Check sheet for the modelled part. Datum: model origin and axes. Units: mm. Face numbers are marked on the shaded views. A direction names the side the tool comes from. Round coordinates to 2 decimals unless told otherwise and drop trailing zeros. Write each loop counter-clockwise with the first axis right and the second up, starting at its lowest first coordinate (ties: lowest second). Pieces come first, ordered by that corner, then holes.
Item 1: Section check B-B, the plane z = 6.5. Record the cut outline in (x, y) (3 decimals), plus the area to 3 significant figures.
Item 2: Depth check by flat-ended pin: pin 1 (8 mm diameter, centred on y = 4, z = 5, fed in from +X) (3 decimals); pin 2 (1.5 mm diameter, centred on y = 15, z = 29, fed in from -X); pin 3 (2 mm diameter, centred on x = 37, z = 50, fed in from +Y). Enter the tip coordinate at first touch or a pass-through.
Item 3: Release check for a two-part mould opening along X. For the marked faces 5, 6 and 7 record: pulls with the +X half, pulls with the -X half, needs draft (parallel to the pull), parting line crosses it, or undercut.
Item 4: Section check D-D, the plane z = 18.5. Record the cut outline in (x, y) (3 decimals).
Item 5: Section check A-A, the plane y = 18. Record the cut outline in (x, z) (3 decimals).
Item 6: Set-up check for the marked faces 1, 2, 3 and 4: record each of +Z, -Z, +X, -X, +Y, -Y from which the full face is reachable in a straight line by a thin tool's end or side.
Item 7: Section check C-C, the plane x = 25. Record the cut outline in (y, z) (3 decimals).
Item 8: Material ranges on line 1 along Y through (x, z) = (68.5, 54); line 2 along Z through (x, y) = (5, 7.5) (3 decimals); line 3 along X through (y, z) = (2, 10) (3 decimals), recorded low to high.
from build123d import *

# Parameters (mm, degrees)
F1_DEPTH = 63.5
F2_DEPTH = 25.4


with BuildPart() as f1:
    # F0 (on Front) → F1 (new body, symmetric)
    with BuildSketch(Plane.XZ):
        Polygon((41.275, -9.525), (41.275, 9.525), (22.225, 9.525), (-41.275, 9.525), (-41.275, -9.525), align=None)
    extrude(amount=F1_DEPTH, both=True)

    # F0 (on Front) → F2 (join, symmetric)
    with BuildSketch(Plane.XZ):
        Polygon((60.325, 61.9252), (60.325, 42.8752), (60.325, 38.1), (85.725, 38.1), (85.547439, 66.675), (60.325, 66.675), align=None)
        with BuildLine():
            Line((22.225, 9.525), (41.275, 9.525))
            Line((41.275, 9.525), (41.275, 27.0002))
            ThreePointArc((41.275, 27.0002), (45.92468, 38.22552), (57.15, 42.8752))
            Line((57.15, 42.8752), (60.325, 42.8752))
            Line((60.325, 42.8752), (60.325, 61.9252))
            Line((60.325, 61.9252), (57.15, 61.9252))
            ThreePointArc((57.15, 61.9252), (32.454296, 51.695904), (22.225, 27.0002))
            Line((22.225, 27.0002), (22.225, 9.525))
        make_face()
    extrude(amount=F2_DEPTH, both=True)


solid = f1.part
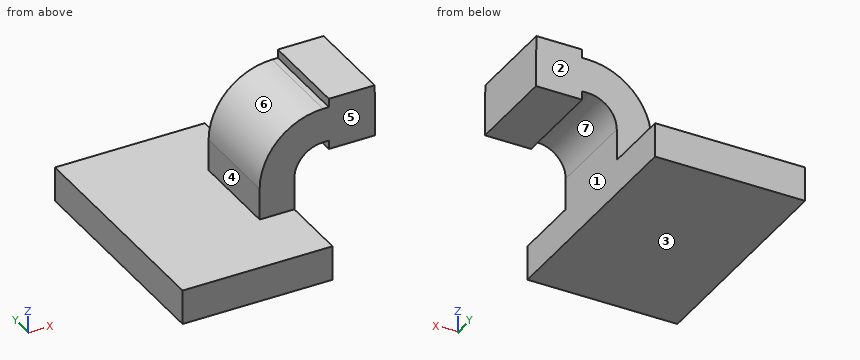
Values found:
1. outline: (-41.275, -63.5) - (41.275, -63.5) - (41.275, 63.5) - (-41.275, 63.5) - close
1. area: 10,500 mm2
2. pin 1: stops at x = 41.275
2. pin 2: stops at x = 22.25
2. pin 3: stops at y = 25.4
3. face 5: needs draft
3. face 6: pulls with the -X half
3. face 7: undercut
4. outline: (22.225, -25.4) - (41.275, -25.4) - (41.275, 25.4) - (22.225, 25.4) - close
5. outline: (-41.275, -9.525) - (41.275, -9.525) - (41.275, 27) arc R15.875 cw to (57.15, 42.875) - (60.325, 42.875) - (60.325, 38.1) - (85.725, 38.1) - (85.547, 66.675) - (60.325, 66.675) - (60.325, 61.925) - (57.15, 61.925) arc R34.925 ccw to (22.225, 27) - (22.225, 9.525) - (-41.275, 9.525) - close
6. face 1: -Z, +X, +Y, -Y
6. face 2: +Z, +X, -X, +Y
6. face 3: -Z, +X, -X, +Y, -Y
6. face 4: +Z, -X, +Y, -Y
7. outline: (-63.5, -9.525) - (63.5, -9.525) - (63.5, 9.525) - (25.4, 9.525) - (25.4, 40.643) - (-25.4, 40.643) - (-25.4, 9.525) - (-63.5, 9.525) - close
8. line 1: y = -25.4 to 25.4
8. line 2: z = -9.525 to 9.525
8. line 3: x = 22.225 to 41.275
